Could you check a few things on this model? Use its own coordinates, in mm. Face numbers are marked on the shaded views. A direction names the side the tool comes from. Coordinates: 2 decimals unless noted, no trailing zeros. Write each loop counter-clockwise with the first axis right and the second up, starting at its lowest first coordinate (ties: lowest second). Pieces come first, ordered by that corner, then holes. Notation, with made-up numbers: (21.5, 81.5) - (68.5, 81.5) arc R9 ccw to (68.5, 97.5) - close; hole circle Ø5 at (-32, 34). An arc over 180 degrees is marked (long way). Answer as a JSON object with one key per item and string values. Group by question number.
1) Please list where these lines run through material, in increasing order: line 1 along Y through (x, z) = (0, 6); line 2 along X through (y, z) = (47, 57.5); line 3 along Z through (x, y) = (16.5, 64.5).
2) If we section it at C-C (z = 13): Write out the boundary of the cut face in (x, y), plus the area to 3 significant figures.
3) If we section it at D-D (x = -20.5): Write out the boundary of the cut face in (y, z), plus the area to 3 significant figures.
4) If we section it at B-B (y = 99): Write out the boundary of the cut face in (x, z).
5) Will these pins go through, and if not, where does the flat tip stop? pin 1 Ø2.5 at (y, z) = (-35, 5.5) entering from -X; pin 2 Ø15.5 at (x, y) = (-1, -22) entering from +Z; pin 3 Ø1.9 at (x, y) = (-12, 52) entering from +Z (3 decimals); pin 4 Ø12 at (x, y) = (-58.5, 81) entering from +Z.
6) If we section it at A-A (x = 0): Write out the boundary of the cut face in (y, z) (3 decimals).
7) On a 3-axis mill with a long thin cutter (end or side, diameter ignored), from which of +Z, -Z, +X, -X, +Y, -Y can I reach the whole of each face in a straight line? I mean the marked faces 1, 2 and 3. Say none if no direction works.
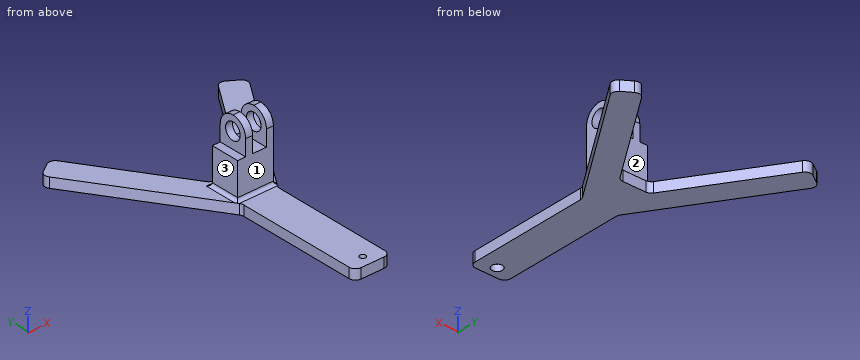
```python
from build123d import *

# Parameters (mm, degrees)
BOSS_EXTRUDE1_DEPTH = 8
SKETCH3_W           = 28.575
SKETCH3_H           = 22.86
BOSS_EXTRUDE2_DEPTH = 52.8
FILLET1_R           = 5.08
SKETCH4_W           = 6.35
SKETCH4_H           = 24.225
SKETCH4_W_2         = 11.049
CUT_EXTRUDE1_DEPTH  = 149.293541653
FILLET3_R           = 11.43
SKETCH5_R           = 6.604
CUT_EXTRUDE2_DEPTH  = 183.273086761
SKETCH7_R           = 4.233333333
CUT_EXTRUDE3_DEPTH  = 5.08
SKETCH8_R           = 2.38125
CUT_EXTRUDE4_DEPTH  = 177.868608292
FILLET7_R           = 2.54


# Some blends are built 0.0001 mm under size
with BuildPart() as part:
    # Sketch1 → Boss-Extrude1 (new body)
    with BuildSketch(Plane.XY):
        Polygon((-11.895004803, 65.589219752), (11.895004803, 65.589219752), (67.084796123, 148.980387954), (82.970813665, 138.466732708), (14.2875, 34.687000521), (14.2875, -66.912999479), (-14.2875, -66.912999479), (-14.2875, 34.687000521), (-82.970813665, 138.466732708), (-67.084796123, 148.980387954), align=None)
    extrude(amount=BOSS_EXTRUDE1_DEPTH)

    # Sketch3 → Boss-Extrude2 (add)
    with BuildSketch(Plane.XY.offset(8)):
        with Locations((0, 50.138110136)):
            Rectangle(SKETCH3_W, SKETCH3_H)
    extrude(amount=BOSS_EXTRUDE2_DEPTH)

    # Fillet1
    fillet1_edges = [part.edges().sort_by_distance(p)[0] for p in [
        (-11.895004803, 65.589219752, 4),
        (11.895004803, 65.589219752, 4),
        (67.084796123, 148.980387954, 4),
        (82.970813665, 138.466732708, 4),
        (14.2875, 34.687000521, 4),
        (14.2875, -66.912999479, 4),
        (-14.2875, -66.912999479, 4),
        (-14.2875, 34.687000521, 4),
        (-82.970813665, 138.466732708, 4),
        (-67.084796123, 148.980387954, 4),
    ]]
    fillet(fillet1_edges, radius=FILLET1_R)

    # Sketch4 → Cut-Extrude1 (cut, through all)
    with BuildSketch(Plane.XZ.offset(-38.708110136)):
        with Locations((-11.1125, 48.6875)):
            Rectangle(SKETCH4_W, SKETCH4_H)
        with Locations((3.175, 48.6875)):
            Rectangle(SKETCH4_W_2, SKETCH4_H)
    extrude(amount=-CUT_EXTRUDE1_DEPTH, mode=Mode.SUBTRACT)

    # Fillet3
    fillet3_edges = [part.edges().sort_by_distance(p)[0] for p in [
        (11.4935, 61.568110136, 60.8),
        (-5.1435, 61.568110136, 60.8),
        (11.4935, 38.708110136, 60.8),
        (-5.1435, 38.708110136, 60.8),
    ]]
    fillet(fillet3_edges, radius=FILLET3_R - 0.0001)  # a hair under: the kernel refuses the full size

    # Sketch5 → Cut-Extrude2 (cut, through all)
    with BuildSketch(Plane.ZY.offset(7.9375)):
        with Locations(Location((49.37, 50.138110136, 0), (0, 0, 270))):
            Circle(SKETCH5_R)
    extrude(amount=-CUT_EXTRUDE2_DEPTH, mode=Mode.SUBTRACT)

    # Sketch7 → Cut-Extrude3 (cut)
    with BuildSketch(Plane(origin=(0, 0, 0), x_dir=(-1, 0, 0), z_dir=(0, 0, -1))):
        with Locations((0, -58.022999479)):
            Circle(SKETCH7_R)
    extrude(amount=-CUT_EXTRUDE3_DEPTH, mode=Mode.SUBTRACT)

    # Sketch8 → Cut-Extrude4 (cut, through all)
    with BuildSketch(Plane(origin=(0, 0, 5.08), x_dir=(-1, 0, 0), z_dir=(0, 0, -1))):
        with Locations((0, -58.022999479)):
            Circle(SKETCH8_R)
    extrude(amount=-CUT_EXTRUDE4_DEPTH, mode=Mode.SUBTRACT)

    # Fillet7
    # the kernel refuses this fillet: 2.54 mm, written as the material it adds along each edge
    with BuildSketch(Plane(origin=(-14.2875, 38.708110136, 8), x_dir=(0, 0, 1), z_dir=(0, 1, 0))) as fillet7_piece_1:
        with BuildLine():
            CenterArc((FILLET7_R, -FILLET7_R), FILLET7_R, 90, 90)
            Line((0, -FILLET7_R), (0, 0))
            Line((0, 0), (FILLET7_R, 0))
        make_face()
    extrude(amount=22.86)
    with BuildSketch(Plane(origin=(14.2875, 38.708110136, 8), x_dir=(0, 0, 1), z_dir=(-1, 0, 0))) as fillet7_piece_2:
        with BuildLine():
            CenterArc((FILLET7_R, -FILLET7_R), FILLET7_R, 90, 90)
            Line((0, -FILLET7_R), (0, 0))
            Line((0, 0), (FILLET7_R, 0))
        make_face()
    extrude(amount=28.575)
    with BuildSketch(Plane(origin=(14.2875, 61.568110136, 8), x_dir=(1, 0, 0), z_dir=(0, -1, 0))) as fillet7_piece_3:
        with BuildLine():
            CenterArc((FILLET7_R, FILLET7_R), FILLET7_R, 180, 90)
            Line((0, FILLET7_R), (0, 0))
            Line((0, 0), (FILLET7_R, 0))
        make_face()
    extrude(amount=22.86)
    with BuildSketch(Plane(origin=(-14.2875, 61.568110136, 8), x_dir=(0, 1, 0), z_dir=(1, 0, 0))) as fillet7_piece_4:
        with BuildLine():
            CenterArc((FILLET7_R, FILLET7_R), FILLET7_R, 180, 90)
            Line((0, FILLET7_R), (0, 0))
            Line((0, 0), (FILLET7_R, 0))
        make_face()
    extrude(amount=28.575)
    with BuildSketch(Plane(origin=(14.2875, 38.708110136, 8), x_dir=(0, 0, 1), z_dir=(-1, 0, 0))) as fillet7_piece_5a_section:
        with BuildLine():
            CenterArc((FILLET7_R, -FILLET7_R), FILLET7_R, 90, 90)
            Line((0, -FILLET7_R), (0, 0))
            Line((0, 0), (FILLET7_R, 0))
        make_face()
    fillet7_piece_5a = extrude(amount=34.925, mode=Mode.PRIVATE)
    fillet7_piece_5a = split(fillet7_piece_5a, bisect_by=Plane(origin=(-14.2875, 38.220078421, 8.626447049), z_dir=(-1, 0, 0)), keep=Keep.TOP, mode=Mode.PRIVATE)
    fillet7_piece_5a = split(fillet7_piece_5a, bisect_by=Plane(origin=(-16.26964909, 37.682006014, 8.626447049), z_dir=(0.833911682022307, 0.5518979131929445, 0)), keep=Keep.TOP, mode=Mode.PRIVATE)
    with BuildSketch(Plane(origin=(-14.2875, 32.358110136, 8), x_dir=(0, 0, 1), z_dir=(0, 1, 0))) as fillet7_piece_5b_section:
        with BuildLine():
            CenterArc((FILLET7_R, -FILLET7_R), FILLET7_R, 90, 90)
            Line((0, -FILLET7_R), (0, 0))
            Line((0, 0), (FILLET7_R, 0))
        make_face()
    fillet7_piece_5b = extrude(amount=29.21, mode=Mode.PRIVATE)
    fillet7_piece_5b = split(fillet7_piece_5b, bisect_by=Plane(origin=(-14.718813993, 38.708110136, 8.659953821), z_dir=(0, -1, 0)), keep=Keep.TOP, mode=Mode.PRIVATE)
    fillet7_piece_5b = split(fillet7_piece_5b, bisect_by=Plane(origin=(-15.49417016, 36.510265873, 8.659953821), z_dir=(0.833911682022307, 0.5518979131929445, 0)), keep=Keep.TOP, mode=Mode.PRIVATE)
    fillet7_piece_5 = fillet7_piece_5a & fillet7_piece_5b
    add(fillet7_piece_5)
    with BuildSketch(Plane(origin=(-14.2875, 38.708110136, 8), x_dir=(0, 0, 1), z_dir=(0, 1, 0))) as fillet7_piece_6a_section:
        with BuildLine():
            CenterArc((FILLET7_R, -FILLET7_R), FILLET7_R, 90, 90)
            Line((0, -FILLET7_R), (0, 0))
            Line((0, 0), (FILLET7_R, 0))
        make_face()
    fillet7_piece_6a = extrude(amount=29.21, mode=Mode.PRIVATE)
    fillet7_piece_6a = split(fillet7_piece_6a, bisect_by=Plane(origin=(-14.86254359, 61.568110136, 8.57504359), z_dir=(0, 1, 0)), keep=Keep.TOP, mode=Mode.PRIVATE)
    with BuildSketch(Plane(origin=(-20.6375, 61.568110136, 8), x_dir=(0, 1, 0), z_dir=(1, 0, 0))) as fillet7_piece_6b_section:
        with BuildLine():
            CenterArc((FILLET7_R, FILLET7_R), FILLET7_R, 180, 90)
            Line((0, FILLET7_R), (0, 0))
            Line((0, 0), (FILLET7_R, 0))
        make_face()
    fillet7_piece_6b = extrude(amount=34.925, mode=Mode.PRIVATE)
    fillet7_piece_6b = split(fillet7_piece_6b, bisect_by=Plane(origin=(-14.2875, 62.143153727, 8.57504359), z_dir=(-1, 0, 0)), keep=Keep.TOP, mode=Mode.PRIVATE)
    fillet7_piece_6 = fillet7_piece_6a & fillet7_piece_6b
    add(fillet7_piece_6)
    with BuildSketch(Plane(origin=(20.6375, 38.708110136, 8), x_dir=(0, 0, 1), z_dir=(-1, 0, 0))) as fillet7_piece_7a_section:
        with BuildLine():
            CenterArc((FILLET7_R, -FILLET7_R), FILLET7_R, 90, 90)
            Line((0, -FILLET7_R), (0, 0))
            Line((0, 0), (FILLET7_R, 0))
        make_face()
    fillet7_piece_7a = extrude(amount=34.925, mode=Mode.PRIVATE)
    fillet7_piece_7a = split(fillet7_piece_7a, bisect_by=Plane(origin=(14.2875, 38.220078421, 8.626447049), z_dir=(1, 0, 0)), keep=Keep.TOP, mode=Mode.PRIVATE)
    fillet7_piece_7a = split(fillet7_piece_7a, bisect_by=Plane(origin=(16.26964909, 37.682006014, 8.626447049), z_dir=(-0.8339116820223075, 0.5518979131929438, 0)), keep=Keep.TOP, mode=Mode.PRIVATE)
    with BuildSketch(Plane(origin=(14.2875, 61.568110136, 8), x_dir=(1, 0, 0), z_dir=(0, -1, 0))) as fillet7_piece_7b_section:
        with BuildLine():
            CenterArc((FILLET7_R, FILLET7_R), FILLET7_R, 180, 90)
            Line((0, FILLET7_R), (0, 0))
            Line((0, 0), (FILLET7_R, 0))
        make_face()
    fillet7_piece_7b = extrude(amount=29.21, mode=Mode.PRIVATE)
    fillet7_piece_7b = split(fillet7_piece_7b, bisect_by=Plane(origin=(14.718813993, 38.708110136, 8.659953821), z_dir=(0, -1, 0)), keep=Keep.TOP, mode=Mode.PRIVATE)
    fillet7_piece_7b = split(fillet7_piece_7b, bisect_by=Plane(origin=(15.49417016, 36.510265872, 8.659953821), z_dir=(-0.8339116820223075, 0.5518979131929438, 0)), keep=Keep.TOP, mode=Mode.PRIVATE)
    fillet7_piece_7 = fillet7_piece_7a & fillet7_piece_7b
    add(fillet7_piece_7)
    with BuildSketch(Plane(origin=(14.2875, 67.918110136, 8), x_dir=(1, 0, 0), z_dir=(0, -1, 0))) as fillet7_piece_8a_section:
        with BuildLine():
            CenterArc((FILLET7_R, FILLET7_R), FILLET7_R, 180, 90)
            Line((0, FILLET7_R), (0, 0))
            Line((0, 0), (FILLET7_R, 0))
        make_face()
    fillet7_piece_8a = extrude(amount=29.21, mode=Mode.PRIVATE)
    fillet7_piece_8a = split(fillet7_piece_8a, bisect_by=Plane(origin=(14.86254359, 61.568110136, 8.57504359), z_dir=(0, 1, 0)), keep=Keep.TOP, mode=Mode.PRIVATE)
    with BuildSketch(Plane(origin=(-14.2875, 61.568110136, 8), x_dir=(0, 1, 0), z_dir=(1, 0, 0))) as fillet7_piece_8b_section:
        with BuildLine():
            CenterArc((FILLET7_R, FILLET7_R), FILLET7_R, 180, 90)
            Line((0, FILLET7_R), (0, 0))
            Line((0, 0), (FILLET7_R, 0))
        make_face()
    fillet7_piece_8b = extrude(amount=34.925, mode=Mode.PRIVATE)
    fillet7_piece_8b = split(fillet7_piece_8b, bisect_by=Plane(origin=(14.2875, 62.143153727, 8.57504359), z_dir=(1, 0, 0)), keep=Keep.TOP, mode=Mode.PRIVATE)
    fillet7_piece_8 = fillet7_piece_8a & fillet7_piece_8b
    add(fillet7_piece_8)


solid = part.part
```
Here are the results:
{
 "1": {"line 1": "y = -66.91 to -60.4, -55.64 to 65.59", "line 2": "x = -7.94 to -2.35, 8.7 to 14.29", "line 3": "z = 0 to 8"},
 "2": {"outline": "(-14.29, 38.71) - (14.29, 38.71) - (14.29, 61.57) - (-14.29, 61.57) - close", "area": "653 mm²"},
 "3": {"outline": "(44.07, 0) - (78.59, 0) - (78.59, 8) - (44.07, 8) - close", "area": "276 mm²"},
 "4": {"outline": "(-56.85, 0) - (-34.01, 0) - (-34.01, 8) - (-56.85, 8) - close; (34.01, 0) - (56.85, 0) - (56.85, 8) - (34.01, 8) - close"},
 "5": {"pin 1": "stops at x = -14.29", "pin 2": "stops at z = 8", "pin 3": "stops at z = 36.575", "pin 4": "passes through"},
 "6": {"outline": "(-66.913, 0) - (-62.256, 0) - (-62.256, 5.08) - (-60.404, 5.08) - (-60.404, 8) - (-66.913, 8) - close; (-55.642, 5.08) - (-53.79, 5.08) - (-53.79, 0) - (65.589, 0) - (65.589, 8) - (64.108, 8) arc R2.54 cw to (61.568, 10.54) - (61.568, 36.575) - (38.708, 36.575) - (38.708, 10.54) arc R2.54 cw to (36.168, 8) - (-55.642, 8) - close"},
 "7": {"face 1": "+Z, +X, -X, -Y", "face 2": "+Z, +X, -X, +Y", "face 3": "+Z, -X, +Y, -Y"}
}
